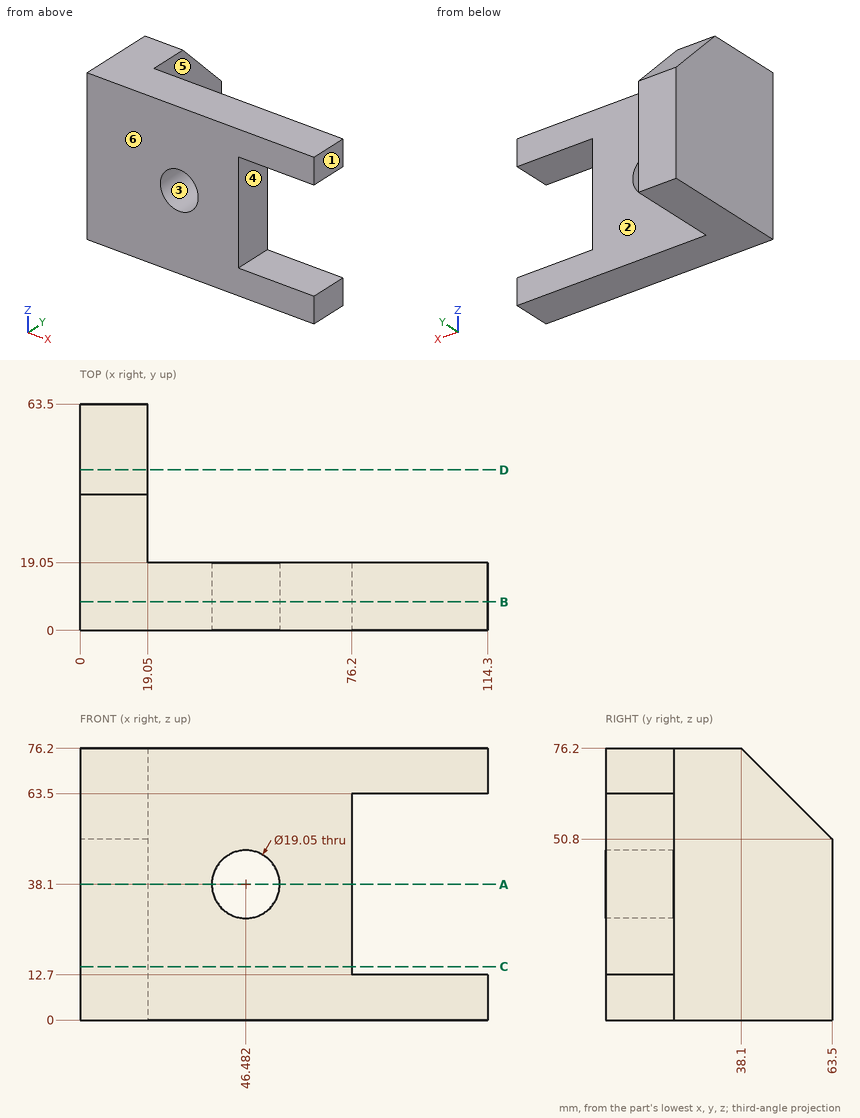
Answer from the drawing. Dimensions are ordinates in mm from the lowest x, y and z of the part. A direction names the side the tool comes from. Give positions to 0.01 mm unless a question says otherwise; leave off trailing zeros. Loops run counter-clockwise (first coordinate to the right, second up) from the corner with the lowest first, then second, coordinate; pieces in that order, holes last. Notation, with made-up numbers: (34, 63) - (50, 63) arc R21 ccw to (50, 100) - close; hole circle Ø2 at (-31.75, -10.5). An arc over 180 degrees is marked (long way). Answer as CSV lines item,"result". Start each with the question number.
Item 1: The mould has two halves that part along X. Classify the marked faces 1, 2 and 3: +X half, -X half, draft (parallel to the pull), parting line (faces both ways), or undercut.
Item 2: A cutting plane is placed at C-C on z = 15. Determine the outline of the cut face in (x, y).
Item 3: A cutting plane is placed at A-A on z = 38.1. Determine the outline of the cut face in (x, y), then the cut area to 3 significant figures.
Item 4: Find the intervals of material crossed by line 1 (X direction, y = 9, z = 38); line 2 (Y direction, x = 26, z = 57.5); line 3 (Z direction, x = 86.5, y = 16), in increasing order. Write a range as from..to.
Item 5: Each of these flat-tipped pins is pushed along its axis until it touches: pin 1 (3 mm diameter, centred on x = 63.5, z = 53, fed in from -Y); pin 2 (5.5 mm diameter, centred on y = 14, z = 49.5, fed in from +X); pin 3 (1 mm diameter, centred on y = 51, z = 41, fed in from +X). Where does it stop, or does it pass through?
Item 6: A cutting plane is placed at D-D on y = 45. Determine the outline of the cut face in (x, z), then the cut area to 3 significant figures.
Item 7: For the marked faces 4, 5 and 6, determine the directions among +Z, -Z, +X, -X, +Y, -Y from which every point of the face is accessible in a straight line to the end or side of a thin tool.
Item 8: A cutting plane is placed at B-B on y = 8. Determine the outline of the cut face in (x, z) (3 decimals), then the cut area to 3 significant figures.
Found:
1,face 1,"+X half"
1,face 2,"draft"
1,face 3,"undercut"
2,outline,"(0, 0) - (76.2, 0) - (76.2, 19.05) - (19.05, 19.05) - (19.05, 63.5) - (0, 63.5) - close"
3,outline,"(0, 0) - (36.96, 0) - (36.96, 19.05) - (19.05, 19.05) - (19.05, 63.5) - (0, 63.5) - close; (56.01, 0) - (76.2, 0) - (76.2, 19.05) - (56.01, 19.05) - close"
3,area,"1,940 mm^2"
4,line 1,"x = 0..36.96, 56.01..76.2"
4,line 2,"y = 0..19.05"
4,line 3,"z = 0..12.7, 63.5..76.2"
5,pin 1,"stops at y = 0"
5,pin 2,"stops at x = 76.2"
5,pin 3,"stops at x = 19.05"
6,outline,"(0, 0) - (19.05, 0) - (19.05, 69.3) - (0, 69.3) - close"
6,area,"1,320 mm^2"
7,face 4,"+X, +Y, -Y"
7,face 5,"+Z, -Z, +X, +Y"
7,face 6,"+Z, -Z, +X, -X, -Y"
8,outline,"(0, 0) - (114.3, 0) - (114.3, 12.7) - (76.2, 12.7) - (76.2, 63.5) - (114.3, 63.5) - (114.3, 76.2) - (0, 76.2) - close; hole circle Ø19.05 at (46.482, 38.1)"
8,area,"6,490 mm^2"
